Input: part model. Units: mm. Frame: model coordinates. Give positions to 0.01 mm unless a question says otherwise; leave off trailing zeros. Loops run counter-clockwise (first coordinate to the right, second up) from the corner with the lowest first, then second, coordinate; pieces in that order, holes last. Notation, with made-up numbers: (-16.5, 86) -> (21.5, 86) arc R17 ccw to (21.5, 111) -> close; hole circle Ø6 at (58.25, 46). An arc over 180 degrees is marked (long way). Use CSV: the item, a comma, the result in double quotes.
```python
from build123d import *

# Parameters (mm, degrees)
SKETCH_1_W          = 50.4
SKETCH_1_H          = 5
SKETCH_1_R          = 1
EXTRUDE_1_DEPTH     = 2
CUT_EXTRUDE_START   = 2
SKETCH_1_8_R        = 1.75
CUT_EXTRUDE_2_DEPTH = 1


with BuildPart() as part:
    # 草图1 → 凸台-拉伸1 (new body)
    with BuildSketch(Plane.XY):
        with Locations((25.2, -2.5)):
            Rectangle(SKETCH_1_W, SKETCH_1_H)
        with Locations((3, -2.5)):
            Circle(SKETCH_1_R, mode=Mode.SUBTRACT)
        with Locations((47.4, -2.5)):
            Circle(SKETCH_1_R, mode=Mode.SUBTRACT)
    extrude(amount=EXTRUDE_1_DEPTH)

    # 草图1<8> → 切除-拉伸2 (cut)
    with BuildSketch(Plane.XY.offset(CUT_EXTRUDE_START)):
        with Locations(Location((3, -2.5, 0), (0, 0, 180))):
            Circle(SKETCH_1_8_R)
        with Locations(Location((47.4, -2.5, 0), (0, 0, 180))):
            Circle(SKETCH_1_8_R)
    extrude(amount=-CUT_EXTRUDE_2_DEPTH, mode=Mode.SUBTRACT)


solid = part.part
```
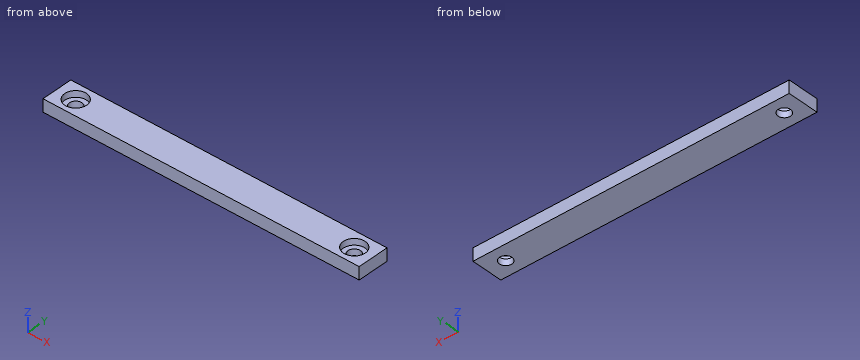
1) Section query B-B (x = 47.4). Return loops of the section in (y, z), then the cut area to 3 significant figures.
From the geometry:
outline,"(-5, 0) -> (-3.5, 0) -> (-3.5, 1) -> (-4.25, 1) -> (-4.25, 2) -> (-5, 2) -> close; (-1.5, 0) -> (0, 0) -> (0, 2) -> (-0.75, 2) -> (-0.75, 1) -> (-1.5, 1) -> close"
area,"4.50 mm^2"
2) Ray query, line 1 (X direction, y = -2.5, z = 1.7); line 2 (Y direction, x = 3, z = 1.35); line 3 (Y direction, x = 3, z = 0.7). Return the intervals inside material, ascending.
From the geometry:
line 1,"x = 0 to 1.25, 4.75 to 45.65, 49.15 to 50.4"
line 2,"y = -5 to -4.25, -0.75 to 0"
line 3,"y = -5 to -3.5, -1.5 to 0"
3) Section query A-A (y = -2.5). Return loops of the section in (x, z), then the cut area to 3 significant figures.
From the geometry:
outline,"(0, 0) -> (2, 0) -> (2, 1) -> (1.25, 1) -> (1.25, 2) -> (0, 2) -> close; (4, 0) -> (46.4, 0) -> (46.4, 1) -> (45.65, 1) -> (45.65, 2) -> (4.75, 2) -> (4.75, 1) -> (4, 1) -> close; (48.4, 0) -> (50.4, 0) -> (50.4, 2) -> (49.15, 2) -> (49.15, 1) -> (48.4, 1) -> close"
area,"89.8 mm^2"
4) Section query C-C (z = 0.3). Return loops of the section in (x, y).
From the geometry:
outline,"(0, -5) -> (50.4, -5) -> (50.4, 0) -> (0, 0) -> close; hole circle Ø2 at (3, -2.5); hole circle Ø2 at (47.4, -2.5)"
